Read the model definition and answer for the solid it produces. Units are mm, in the model's axes. A direction names the side the tool comes from. Give positions to 0.01 mm unless a question says otherwise; leave off trailing zeros. Order: outer loops, then holes, each group sorted by start corner. A loop starts at its lowest first (then second) coordinate and runs counter-clockwise, first axis right, second up.
Item 1: A cutting plane is placed at C-C (z = 17). Write down the section's boundary in (x, y).
Item 2: Given pin 1 Ø5 at (x, z) = (-23.5, 15.5) entering from +Y; pin 2 Ø7.5 at (x, z) = (135, 18) entering from -Y; pin 3 Ø5.5 at (x, y) = (52, -77.5) entering from -Z, each flat-ended and moving along its own axis, determine where each tip first touches the part or whether it passes through.
Item 3: A cutting plane is placed at D-D (y = 81). Write down the section's boundary in (x, z) (3 decimals).
Item 4: The mould has two halves that part along Y. Classify faces 1 (the face through (44, 93.331, 18)), 2 (the face through (38, 93.331, 83)), 3 (the face through (44, -81, 76.2)), 4 (the face through (40, -90.819, 11)): +Y half, -Y half, draft (parallel to the pull), parting line (faces both ways), or undercut.
Item 5: A cutting plane is placed at B-B (z = 70.5). Write down the section's boundary in (x, y).
Item 6: A cutting plane is placed at A-A (x = -59). Write down the section's boundary in (y, z) (3 decimals).
Item 7: Which of the six approach directions +Z, -Z, +X, -X, +Y, -Y give full straight-line access (tool end or side, diameter ignored) to faces 5 (the face through (44, 103, 76.2)), 6 (the face through (44, 103, 12.7)), 7 (the face through (44, 12, 22.225)), 8 (the face through (38, -71.769, 18))?
Item 8: Find the intervals of material crossed by line 1 along X through (y, z) = (28.5, 58.5); line 2 along Y through (x, z) = (86, 78.5); line 3 along Z through (x, y) = (123, -72.5), in increasing order.
from build123d import *

# Parameters (mm, degrees)
F0_W     = 431.8
F0_H     = 203.2
F1_DEPTH = 88.9
F2_W     = 419.1
F2_H     = 53.975
F3_DEPTH = 203.2
F4_W     = 419.1
F4_H     = 165.1
F5_DEPTH = 12.7
F6_W     = 419.1
F6_H     = 9.525
F7_DEPTH = 19.05
F8_W     = 419.1
F8_H     = 9.525
F9_DEPTH = 19.05


with BuildPart() as f1:
    # F0 (on Top) → F1 (new body)
    with BuildSketch(Plane.XY):
        with Locations((40.765872, 10.780569)):
            Rectangle(F0_W, F0_H)
    extrude(amount=F1_DEPTH)

    # F2 (on face) → F3 (cut, through all)
    with BuildSketch(Plane(origin=(0, 112.380569, 0), x_dir=(-1, 0, 0), z_dir=(0, 1, 0))):
        with Locations((-40.765872, 49.2125)):
            Rectangle(F2_W, F2_H)
    extrude(amount=-F3_DEPTH, mode=Mode.SUBTRACT)

    # F4 (on face) → F5 (cut, through all)
    with BuildSketch(Plane.XY.offset(88.9)):
        with Locations((40.765872, 10.780569)):
            Rectangle(F4_W, F4_H)
    extrude(amount=-F5_DEPTH, mode=Mode.SUBTRACT)

    # F6 (on face) → F7 (cut)
    with BuildSketch(Plane(origin=(0, 112.380569, 0), x_dir=(-1, 0, 0), z_dir=(0, 1, 0))):
        with Locations((-40.765872, 17.4625)):
            Rectangle(F6_W, F6_H)
    extrude(amount=-F7_DEPTH, mode=Mode.SUBTRACT)

    # F8 (on face) → F9 (cut)
    with BuildSketch(Plane.XZ.offset(90.819431)):
        with Locations((40.765872, 17.4625)):
            Rectangle(F8_W, F8_H)
    extrude(amount=-F9_DEPTH, mode=Mode.SUBTRACT)


solid = f1.part
Response values:
1. outline: (-175.13, -90.82) - (-168.78, -90.82) - (-168.78, -71.77) - (250.32, -71.77) - (250.32, -90.82) - (256.67, -90.82) - (256.67, 112.38) - (250.32, 112.38) - (250.32, 93.33) - (-168.78, 93.33) - (-168.78, 112.38) - (-175.13, 112.38) - close
2. pin 1: stops at y = 93.33
2. pin 2: stops at y = -71.77
2. pin 3: stops at z = 0
3. outline: (-175.134, 0) - (256.666, 0) - (256.666, 88.9) - (250.316, 88.9) - (250.316, 22.225) - (-168.784, 22.225) - (-168.784, 88.9) - (-175.134, 88.9) - close
4. face 1: +Y half
4. face 2: undercut
4. face 3: draft
4. face 4: -Y half
5. outline: (-175.13, -90.82) - (-168.78, -90.82) - (-168.78, 112.38) - (-175.13, 112.38) - close; (250.32, -90.82) - (256.67, -90.82) - (256.67, 112.38) - (250.32, 112.38) - close
6. outline: (-90.819, 0) - (112.381, 0) - (112.381, 12.7) - (93.331, 12.7) - (93.331, 22.225) - (-71.769, 22.225) - (-71.769, 12.7) - (-90.819, 12.7) - close; (-90.819, 76.2) - (-71.769, 76.2) - (-71.769, 88.9) - (-90.819, 88.9) - close; (93.331, 76.2) - (112.381, 76.2) - (112.381, 88.9) - (93.331, 88.9) - close
7. face 5: +Y, -Y
7. face 6: +Y
7. face 7: +Z, +Y, -Y
7. face 8: -Y
8. line 1: x = -175.13 to -168.78, 250.32 to 256.67
8. line 2: y = -90.82 to -71.77, 93.33 to 112.38
8. line 3: z = 0 to 12.7, 76.2 to 88.9
